```python
from build123d import *

# Parameters (mm, degrees)
SKETCH_1_R          = 1.25
EXTRUDE_1_DEPTH     = 8
FILLET_1_R          = 4
SKETCH_2_R          = 1.25
CUT_EXTRUDE_1_DEPTH = 10
SKETCH_3_R          = 1.25
CUT_EXTRUDE_2_DEPTH = 67


with BuildPart() as part:
    # 草图1 → 凸台-拉伸1 (new body)
    # profile 1 of 2: a face of its own
    with BuildSketch(Plane.XY):
        Polygon((0, 46), (0, 23), (14, 23), (14, 30), (60, 30), (60, 46), align=None)
        with Locations((17, 35.5)):
            Circle(SKETCH_1_R, mode=Mode.SUBTRACT)
        with Locations((42, 35.5)):
            Circle(SKETCH_1_R, mode=Mode.SUBTRACT)
    # profile 2 of 2: a face of its own
    with BuildSketch(Plane.XY):
        Polygon((14, 23), (0, 23), (0, 0), (60, 0), (60, 16), (14, 16), align=None)
        with Locations((17, 10.5)):
            Circle(SKETCH_1_R, mode=Mode.SUBTRACT)
        with Locations((42, 10.5)):
            Circle(SKETCH_1_R, mode=Mode.SUBTRACT)
    extrude(amount=EXTRUDE_1_DEPTH)

    # 圆角1
    fillet_1_edges = [part.edges().sort_by_distance(p)[0] for p in [
        (0, 46, 4),
        (60, 46, 4),
        (60, 30, 4),
        (14, 30, 4),
        (14, 16, 4),
        (60, 16, 4),
        (60, 0, 4),
        (0, 0, 4),
    ]]
    fillet(fillet_1_edges, radius=FILLET_1_R)

    # 草图2 → 切除-拉伸1 (cut)
    with BuildSketch(Plane.XY.offset(8)):
        with Locations((17, 3)):
            Circle(SKETCH_2_R)
        with Locations((37, 3)):
            Circle(SKETCH_2_R)
        with Locations((37, 43)):
            Circle(SKETCH_2_R)
        with Locations((17, 43)):
            Circle(SKETCH_2_R)
    extrude(amount=-CUT_EXTRUDE_1_DEPTH, mode=Mode.SUBTRACT)

    # 草图3 → 切除-拉伸2 (cut)
    with BuildSketch(Plane(origin=(0, 46, 0), x_dir=(1, 0, 0), z_dir=(0, 1, 0))):
        with Locations(Location((27, -3, 0), (0, 0, 270))):
            Circle(SKETCH_3_R)
        with Locations(Location((47, -3, 0), (0, 0, 270))):
            Circle(SKETCH_3_R)
    extrude(amount=-CUT_EXTRUDE_2_DEPTH, mode=Mode.SUBTRACT)


solid = part.part
```
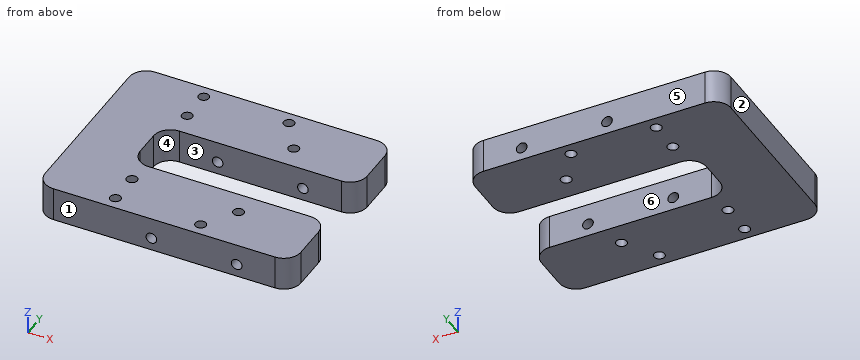
Model file for the job. Use its own axes, mm. Face numbers are marked on the shaded views. A direction names the side the tool comes from. Coordinates: 2 decimals unless noted, no trailing zeros. Order: outer loops, then holes, each group sorted by start corner. A loop starts at its lowest first (then second) coordinate and runs counter-clockwise, first axis right, second up. Notation, with made-up numbers: (-14.5, 55) - (23.5, 55) arc R30 ccw to (23.5, 88) - close; hole circle Ø3 at (-30.75, 16). An arc over 180 degrees is marked (long way). Return JSON: item names as keys, results as strings. Group by question number.
1) Saw through at D-D, the plane y = 38. Write the cut outline in (x, z), plus the area to 3 significant figures.
2) Saw through at A-A, the plane y = 10.5. Write the cut outline in (x, z), plus the area to 3 significant figures.
3) Flat gauge pin, fed straight in: P1, Ø1.8, axis at y = 22, z = 5.5, coming from the +X side. Where does the tip first touch, or does it go through?
4) Saw through at C-C, the plane z = 7. Count the separate pieces of the cut face and the enclosed holes in it, plus the area to 3 significant figures.
5) Probe line 1 (Y direction, x = 37, z = 2.75); line 2 (Y direction, x = 29, z = 3); line 3 (X direction, y = 5.75, z = 3). List the from-to ranges inside material, lowest first. Write a range as from..to.
6) Mould opens along Y. For the marked faces 1, 2, 3 and 4 say: released by +Y, released by -Y, zero draft, split by the parting line, or undercut.
7) Saw through at B-B, the plane x = 37. Write the cut outline in (y, z), plus the area to 3 significant figures.
8) Tool access for the marked faces 5 and 6: list every direction of +Z, -Z, +X, -X, +Y, -Y with a clear straight run to the whole face (end or side of a thin tool).
Values found:
{
 "1": {"outline": "(0, 0) - (60, 0) - (60, 8) - (0, 8) - close; hole circle Ø2.5 at (27, 3); hole circle Ø2.5 at (47, 3)", "area": "470 mm²"},
 "2": {"outline": "(0, 0) - (15.75, 0) - (15.75, 8) - (0, 8) - close; (18.25, 0) - (40.75, 0) - (40.75, 8) - (18.25, 8) - close; (43.25, 0) - (60, 0) - (60, 8) - (43.25, 8) - close; hole circle Ø2.5 at (27, 3); hole circle Ø2.5 at (47, 3)", "area": "430 mm²"},
 "3": {"P1": "stops at x = 14"},
 "4": {"separate pieces": "1", "enclosed holes": "8", "area": "2,060 mm²"},
 "5": {"line 1": "y = 0..1.75, 4.25..16, 30..41.75, 44.25..46", "line 2": "y = 0..16, 30..46", "line 3": "x = 0..25.75, 28.25..45.75, 48.25..60"},
 "6": {"face 1": "released by -Y", "face 2": "zero draft", "face 3": "undercut", "face 4": "undercut"},
 "7": {"outline": "(0, 0) - (1.75, 0) - (1.75, 8) - (0, 8) - close; (4.25, 0) - (16, 0) - (16, 8) - (4.25, 8) - close; (30, 0) - (41.75, 0) - (41.75, 8) - (30, 8) - close; (44.25, 0) - (46, 0) - (46, 8) - (44.25, 8) - close", "area": "216 mm²"},
 "8": {"face 5": "+Z, -Z, +X, -X, +Y", "face 6": "+Z, -Z, +X"}
}
